The listing builds one solid part. Answer for the finished solid, in the listing's coordinates (mm). Face numbers are marked on the shaded views. A direction names the side the tool comes from. Round coordinates to 2 decimals unless told otherwise and drop trailing zeros. Write each loop counter-clockwise with the first axis right and the second up, starting at its lowest first coordinate (ties: lowest second). Pieces come first, ordered by that corner, then holes. Notation, with made-up numbers: (70.25, 41) - (113.25, 41) arc R23 ccw to (113.25, 79) - close; hole circle Ø6 at (55.5, 36). An arc over 180 degrees is marked (long way). Use a Markdown table: item, result. Add a question column.
1) Determine the mould class of the marked faces 1, 2, 3 and 4 for opening direction X: +X half, -X half, draft (parallel to the pull), parting line (faces both ways), or undercut.
2) A cutting plane is placed at A-A (x = 4.25). Give the vertices of the cut face in (y, z), then the cut area to 3 significant figures.
3) Find the intervals of material crossed by probe 1 along Y at (x, z) = (4, 2.6); probe 2 along X at (y, z) = (-0.75, 0.75); probe 3 along Y at (x, z) = (5.5, 1.65), in increasing order. Write a range as from..to.
4) Each of these flat-tipped pins is pushed along its axis until it touches: P1, Ø1.4, axis at y = 0, z = 3, coming from the -X side; P2, Ø1, axis at x = 4.5, z = 2, coming from the -Y side; P3, Ø1.8, axis at y = -1, z = 1, coming from the -X side. Where does it stop, or does it pass through?
5) A cutting plane is placed at B-B (y = -0.5). Give the vertices of the cut face in (x, z).
6) A tool of negligible diameter and unlimited length cuts with its end or side. For the marked faces 5, 6 and 7, from which of +Z, -Z, +X, -X, +Y, -Y can it reach the whole face along a straight path? Write none if from no direction.
7) A cutting plane is placed at D-D (x = 1.25). Give the vertices of the cut face in (y, z).
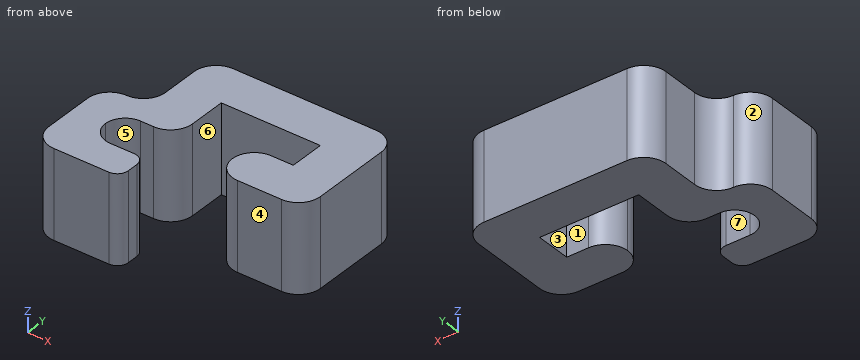
```python
from build123d import *

# Parameters (mm, degrees)
F1_DEPTH = 4
F2_R     = 0.99999
F3_R     = 0.89999
F4_R     = 0.5


# Not quite as in the source:
# - a fillet or chamfer is up to 0.001 mm smaller than in the source, because OpenCascade refuses the exact size


with BuildPart() as f1:
    # F0 (on Top) → F1 (new body)
    with BuildSketch(Plane.XY):
        Polygon((0, -2.7), (0, 0), (4.5, 0), (4.5, -1.6), (2.5, -1.6), (2.5, -3.6), (6.5, -3.6), (6.5, 2), (-2, 2), (-2, -1.7), (-4, -1.7), (-4, -6), (0, -6), (0, -4.5), (-2.5, -4.5), (-2.5, -2.7), align=None)
    extrude(amount=F1_DEPTH)

    # F2 (radius 1 in the source; OpenCascade refuses exactly that, so slightly less here)
    f2_edges = [f1.edges().sort_by_distance(p)[0] for p in [
        (6.5, -3.6, 2),
        (6.5, 2, 2),
        (-2, 2, 2),
        (-2, -1.7, 2),
        (-4, -1.7, 2),
        (-4, -6, 2),
        (2.5, -3.6, 2),
        (0, -2.7, 2),
        (2.5, -1.6, 2),
    ]]
    fillet(f2_edges, radius=F2_R)

    # F3 (radius 0.9 in the source; OpenCascade refuses exactly that, so slightly less here)
    f3_edges = [f1.edges().sort_by_distance(p)[0] for p in [
        (-2.5, -2.7, 2),
        (-2.5, -4.5, 2),
    ]]
    fillet(f3_edges, radius=F3_R)

    # F4
    f4_edges = [f1.edges().sort_by_distance(p)[0] for p in [
        (0, -6, 2),
        (0, -4.5, 2),
    ]]
    fillet(f4_edges, radius=F4_R)


solid = f1.part
```
Entries:
| question | item | result |
|---|---|---|
| 1 | face 1 | undercut |
| 1 | face 2 | -X half |
| 1 | face 3 | undercut |
| 1 | face 4 | draft |
| 2 | outline | (-3.6, 0) - (-1.6, 0) - (-1.6, 4) - (-3.6, 4) - close; (0, 0) - (2, 0) - (2, 4) - (0, 4) - close |
| 2 | area | 16.0 mm² |
| 3 | probe 1 | y = -3.6..-1.6, 0..2 |
| 3 | probe 2 | x = -2..0, 4.5..6.5 |
| 3 | probe 3 | y = -3.6..2 |
| 4 | P1 | stops at x = -2 |
| 4 | P2 | stops at y = -3.6 |
| 4 | P3 | stops at x = -3.6 |
| 5 | outline | (-2, 0) - (0, 0) - (0, 4) - (-2, 4) - close; (4.5, 0) - (6.5, 0) - (6.5, 4) - (4.5, 4) - close |
| 6 | face 5 | +Z, -Z |
| 6 | face 6 | +Z, -Z, -Y |
| 6 | face 7 | +Z, -Z, +X |
| 7 | outline | (0, 0) - (2, 0) - (2, 4) - (0, 4) - close |
